For this review, take the finished solid that the model builds, in its own axes (mm). Give positions to 0.01 mm unless a question says otherwise; leave off trailing zeros. Loops run counter-clockwise (first coordinate to the right, second up) from the corner with the lowest first, then second, coordinate; pieces in that order, holes last. Notation, with made-up numbers: (25.5, -8) - (46.5, -8) arc R27 ccw to (46.5, 9) - close; hole circle Ø5 at (-29.75, 37). An arc over 180 degrees is marked (long way). Answer as CSV lines item,"result".
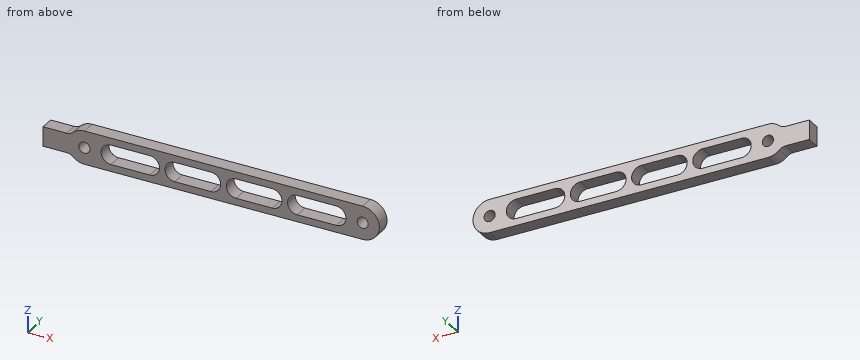
from build123d import *

# Parameters (mm, degrees)
SKETCH1_R           = 4
SKETCH1_W           = 42
SKETCH1_H           = 14
SKETCH1_W_2         = 40
BOSS_EXTRUDE1_DEPTH = 10
FILLET1_R           = 7


with BuildPart() as part:
    # Sketch1 → Boss-Extrude1 (new body)
    with BuildSketch(Plane(origin=(0, 0, 0), x_dir=(1, 0, 0), z_dir=(0, 1, 0))):
        with BuildLine():
            Line((-200, 12), (0, 12))
            ThreePointArc((0, 12), (12, 0), (0, -12))
            Line((0, -12), (-200, -12))
            ThreePointArc((-200, -12), (-205.477225575, -10.677078252), (-209.746794345, -7))
            Line((-209.746794345, -7), (-229.746794345, -7))
            Line((-229.746794345, -7), (-229.746794345, 7))
            Line((-229.746794345, 7), (-209.746794345, 7))
            ThreePointArc((-209.746794345, 7), (-205.477225575, 10.677078252), (-200, 12))
        make_face()
        with Locations(Location((-200, 0, 0), (0, 0, 270))):
            Circle(SKETCH1_R, mode=Mode.SUBTRACT)
        with Locations(Location((0, 0, 0), (0, 0, 270))):
            Circle(SKETCH1_R, mode=Mode.SUBTRACT)
        with Locations((-167, 0)):
            Rectangle(SKETCH1_W, SKETCH1_H, mode=Mode.SUBTRACT)
        with Locations((-122, 0)):
            Rectangle(SKETCH1_W_2, SKETCH1_H, mode=Mode.SUBTRACT)
        with Locations((-78, 0)):
            Rectangle(SKETCH1_W_2, SKETCH1_H, mode=Mode.SUBTRACT)
        with Locations((-33, 0)):
            Rectangle(SKETCH1_W, SKETCH1_H, mode=Mode.SUBTRACT)
    extrude(amount=BOSS_EXTRUDE1_DEPTH)

    # Fillet1
    fillet1_edges = [part.edges().sort_by_distance(p)[0] for p in [
        (-142, 5, -7),
        (-98, 5, -7),
        (-54, 5, -7),
        (-58, 5, -7),
        (-12, 5, -7),
        (-102, 5, -7),
        (-146, 5, -7),
        (-146, 5, 7),
        (-102, 5, 7),
        (-58, 5, 7),
        (-12, 5, 7),
        (-54, 5, 7),
        (-98, 5, 7),
        (-142, 5, 7),
        (-188, 5, 7),
        (-188, 5, -7),
        (-209.746794345, 5, 7),
        (-209.746794345, 5, -7),
    ]]
    fillet(fillet1_edges, radius=FILLET1_R - 0.0001)  # a hair under: the kernel refuses the full size


solid = part.part
1) Insertion check: P1, Ø1.5, axis at x = -121.5, z = -6, coming from the -Y side; P2, Ø4, axis at y = 5.5, z = -7.5, coming from the +X side; P3, Ø1.5, axis at y = 6, z = 5, coming from the +X side; P4, Ø3, axis at x = -220.5, y = 3, coming from the +Z side. Each pin has a flat end and moves straight along its axis. Give the tip position at first contact, or say it passes through.
From the geometry:
P1,"passes through"
P2,"stops at x = 10.67"
P3,"stops at x = 11.22"
P4,"stops at z = 7"
2) Consider section A-A on x = -27.5. Write out the cut boundary in (y, z), and give its area (3 significant figures).
From the geometry:
outline,"(0, -12) - (10, -12) - (10, -7) - (0, -7) - close; (0, 7) - (10, 7) - (10, 12) - (0, 12) - close"
area,"100 mm^2"
3) Wall thickness on line 1 (Z direction, x = -131.5, y = 2); line 2 (X direction, y = 5.75, z = 4.25); line 3 (X direction, y = 9.5, z = 11): over which ranges is each line inside the solid? List them lowest first. Write a range as from..to.
From the geometry:
line 1,"z = -12..-7, 7..12"
line 2,"x = -229.75..-186.56, -147.44..-140.56, -103.44..-96.56, -59.44..-52.56, -13.44..11.22"
line 3,"x = -204.8..4.8"
4) Consider section B-B on y = 7.75. Count the separate pieces of the cut face and the enclosed holes in it, and give its area (3 significant figures).
From the geometry:
separate pieces,"1"
enclosed holes,"6"
area,"3,280 mm^2"
